Could you check a few things on this model? Use its own coordinates, in mm. A direction names the side the tool comes from. Give positions to 0.01 mm unless a question says otherwise; leave off trailing zeros. Loops run counter-clockwise (first coordinate to the right, second up) from the corner with the lowest first, then second, coordinate; pieces in that order, holes last. Notation, with made-up numbers: (83, 73.25) -> (136, 73.25) arc R31 cw to (136, 98.25) -> close; hole circle Ø2 at (-10.75, 16). An arc over 180 degrees is marked (long way). Write item = value, one per line. Start each with the question number.
1) On a 3-axis mill with a long thin cutter (end or side, diameter ignored), from which of +Z, -Z, +X, -X, +Y, -Y can I reach the whole of each face in a straight line? I mean faces 1 (the face through (21.596, 5.982, 5.479)), 2 (the face through (-1, 68.522, 3)). Say none if no direction works.
2) I want a section at B-B (x = 20). List the corners of the cut face in (y, z) for me, and give its area (3 significant figures).
3) I need wall thicknesses on probe 1 along Y at (x, z) = (0, 5.2); probe 2 along Y at (x, z) = (30.5, 5); probe 3 along X at (y, z) = (7, 4.5). Which ranges of each line are inside material? Lowest first, please. Write a range as from..to.
4) I'm going to push a flat-ended pin straight in: pin 1 Ø10 at (x, y) = (-31, 51) entering from +Z. Where does the tip first touch, or does it pass through?
5) If we mould it in two halves opening along Y, with no side actions, what happens to faces 3 (the face through (-35, 16, 4)), 4 (the face through (-1, 34, 0)), 5 (the face through (-1, -1.478, 3))? For each: +Y half, -Y half, draft (parallel to the pull), parting line (faces both ways), or undercut.
6) I want a section at D-D (x = -34.5). List the corners of the cut face in (y, z) for me.
7) I want a section at C-C (y = 21). List the corners of the cut face in (x, z) for me, and give its area (3 significant figures).
8) I want a section at A-A (y = 59). List the corners of the cut face in (x, z) for me, and give its area (3 significant figures).
from build123d import *

# Parameters (mm, degrees)
F0_W     = 110
F0_H     = 70
F0_R     = 16.5
F1_DEPTH = 7
F2_DEPTH = 4


with BuildPart() as f1:
    # F0 (on Top) → F1 (new body)
    with BuildSketch(Plane.XY):
        with Locations((0, 33.521559)):
            Rectangle(F0_W, F0_H)
        with Locations((-34.310443, 16.02208)):
            Circle(F0_R, mode=Mode.SUBTRACT)
        with Locations((0.189557, 16.02208)):
            Circle(F0_R, mode=Mode.SUBTRACT)
        with Locations((34.689557, 16.02208)):
            Circle(F0_R, mode=Mode.SUBTRACT)
        with Locations((-34.5, 50.521559)):
            Circle(F0_R, mode=Mode.SUBTRACT)
        with Locations((0, 50.521559)):
            Circle(F0_R, mode=Mode.SUBTRACT)
        with Locations((34.5, 50.521559)):
            Circle(F0_R, mode=Mode.SUBTRACT)
    extrude(amount=F1_DEPTH)

    # F0 (on Top) → F2 (join)
    with BuildSketch(Plane.XY):
        with Locations((-34.5, 50.521559)):
            Circle(F0_R)
        with Locations((0, 50.521559)):
            Circle(F0_R)
        with Locations((34.5, 50.521559)):
            Circle(F0_R)
        with Locations((34.689557, 16.02208)):
            Circle(F0_R)
        with Locations((0.189557, 16.02208)):
            Circle(F0_R)
        with Locations((-34.310443, 16.02208)):
            Circle(F0_R)
    extrude(amount=F2_DEPTH)


solid = f1.part
Answer list:
q1.face_1 = +Z
q1.face_2 = +Z, -Z, +X, -X, +Y
q2.outline = (-1.48, 0) -> (68.52, 0) -> (68.52, 7) -> (58.4, 7) -> (58.4, 4) -> (42.65, 4) -> (42.65, 7) -> (23.54, 7) -> (23.54, 4) -> (8.51, 4) -> (8.51, 7) -> (-1.48, 7) -> close
q2.area = 398 mm^2
q3.probe_1 = -1.48..-0.48, 32.52..34.02, 67.02..68.52
q3.probe_2 = -1.48..0.06, 31.98..34.51, 66.53..68.52
q3.probe_3 = -55..-48.13, -20.5..-13.63, 14..20.87, 48.5..55
q4.pin_1 = 4
q5.face_3 = undercut
q5.face_4 = draft
q5.face_5 = -Y half
q6.outline = (-1.48, 0) -> (68.52, 0) -> (68.52, 7) -> (67.02, 7) -> (67.02, 4) -> (34.02, 4) -> (34.02, 7) -> (32.52, 7) -> (32.52, 4) -> (-0.48, 4) -> (-0.48, 7) -> (-1.48, 7) -> close
q7.outline = (-55, 0) -> (55, 0) -> (55, 7) -> (50.42, 7) -> (50.42, 4) -> (18.96, 4) -> (18.96, 7) -> (15.92, 7) -> (15.92, 4) -> (-15.54, 4) -> (-15.54, 7) -> (-18.58, 7) -> (-18.58, 4) -> (-50.04, 4) -> (-50.04, 7) -> (-55, 7) -> close
q7.area = 487 mm^2
q8.outline = (-55, 0) -> (55, 0) -> (55, 7) -> (48.66, 7) -> (48.66, 4) -> (20.34, 4) -> (20.34, 7) -> (14.16, 7) -> (14.16, 4) -> (-14.16, 4) -> (-14.16, 7) -> (-20.34, 7) -> (-20.34, 4) -> (-48.66, 4) -> (-48.66, 7) -> (-55, 7) -> close
q8.area = 515 mm^2
